Model file for the job. Use its own axes, mm. A direction names the side the tool comes from. Give positions to 0.01 mm unless a question says otherwise; leave off trailing zeros. Loops run counter-clockwise (first coordinate to the right, second up) from the corner with the lowest first, then second, coordinate; pieces in that order, holes last. Notation, with made-up numbers: M -11,70.5 L -4,70.5 A25 cw -4,97.5 Z; hole C 2.25,-35.5 d1. An arc over 180 degrees is marked long. Answer in a Markdown table with one row per item.
```python
from build123d import *

# Parameters (mm, degrees)
F0_R     = 38.47128
F0_R_2   = 20.373798
F1_DEPTH = 50
F2_DEPTH = 85
F3_DEPTH = 85
F4_DEPTH = 50


with BuildPart() as f1:
    # F0 (on Front) → F1 (new body)
    with BuildSketch(Plane.XZ):
        Circle(F0_R)
        Circle(F0_R_2, mode=Mode.SUBTRACT)
    extrude(amount=F1_DEPTH)

    # F0 (on Front) → F2 (join)
    with BuildSketch(Plane.XZ):
        Circle(F0_R_2)
    extrude(amount=F2_DEPTH)

    # F0 (on Front) → F3 (join)
    with BuildSketch(Plane.XZ):
        Circle(F0_R_2)
    extrude(amount=-F3_DEPTH)

    # F0 (on Front) → F4 (join)
    with BuildSketch(Plane.XZ):
        Circle(F0_R)
        Circle(F0_R_2, mode=Mode.SUBTRACT)
    extrude(amount=-F4_DEPTH)


solid = f1.part
```
(1) Which spindle directions (+Z, -Z, +X, -X, +Y, -Y) get a long thin tool onto all of the face, cutting with end or side? Do faces 1 (the flat face through (0, -85, 0)), 2 (the flat face through (17, 50, -17)), 3 (the flat face through (17, -50, -17)). Say none if no direction does.
Established:
| item | result |
|---|---|
| face 1 | +Z, -Z, +X, -X, -Y |
| face 2 | +Y |
| face 3 | -Y |
(2) Saw through at A-A, the plane x = 0. Give the cut face in (y, z), and give its area (3 significant figures).
Established:
| item | result |
|---|---|
| outline | M -85,-20.37 L -50,-20.37 L -50,-38.47 L 50,-38.47 L 50,-20.37 L 85,-20.37 L 85,20.37 L 50,20.37 L 50,38.47 L -50,38.47 L -50,20.37 L -85,20.37 Z |
| area | 10,500 mm2 |
(3) Saw through at B-B, the plane z = 0. Give the cut face in (x, y), and give its area (3 significant figures).
Established:
| item | result |
|---|---|
| outline | M -38.47,-50 L -20.37,-50 L -20.37,-85 L 20.37,-85 L 20.37,-50 L 38.47,-50 L 38.47,50 L 20.37,50 L 20.37,85 L -20.37,85 L -20.37,50 L -38.47,50 Z |
| area | 10,500 mm2 |
(4) Wall check: L1, parallel to Y at x = 27, z = -16.5; L2, parallel to Z at x = 16, y = -35; L3, parallel to X at y = 28, z = 17.5. Give the ranges that are in metal, low to high.
Established:
| item | result |
|---|---|
| L1 | y = -50 to 50 |
| L2 | z = -34.99 to 34.99 |
| L3 | x = -34.26 to 34.26 |
(5) Saw through at D-D, the plane y = -17.5. Give the cut face in (x, z), and give its area (3 significant figures).
Established:
| item | result |
|---|---|
| outline | C 0,0 d76.94 |
| area | 4,650 mm2 |
(6) Saw through at C-C, the plane y = -60.5. Give the cut face in (x, z).
Established:
| item | result |
|---|---|
| outline | C 0,0 d40.75 |
(7) Flat gauge pins, fed straight in: P1, Ø4, axis at y = -50, z = -23, coming from the +X side; P2, Ø1.5, axis at y = 46.5, z = -9.5, coming from the +X side; P3, Ø8, axis at x = -23.5, z = 27, coming from the -Y side. Where does each tip first touch, or does it go through?
Established:
| item | result |
|---|---|
| P1 | stops at x = 32.23 |
| P2 | stops at x = 37.46 |
| P3 | stops at y = -50 |
